The model under review builds one solid part; all positions refer to its coordinate system, in mm. A direction names the side the tool comes from. Coordinates: 2 decimals unless noted, no trailing zeros. Order: outer loops, then holes, each group sorted by start corner. A loop starts at its lowest first (then second) coordinate and runs counter-clockwise, first axis right, second up. Notation, with made-up numbers: (-29, 37) -> (6, 37) arc R19 ccw to (6, 45) -> close; hole circle Ø2 at (1, -25.5). An arc over 180 degrees is marked (long way). Put each result on its own line as item: value.
from build123d import *

# Parameters (mm, degrees)
SKETCH1_R           = 26.5
BOSS_EXTRUDE1_DEPTH = 3
BOSS_EXTRUDE2_START = 3
SKETCH1_3_R         = 26.5
SKETCH1_3_R_2       = 25
BOSS_EXTRUDE2_DEPTH = 10
CUT_EXTRUDE1_DEPTH  = 39.787884706
SKETCH3_R           = 26.5
SKETCH3_R_2         = 25
BOSS_EXTRUDE3_DEPTH = 10
SKETCH5_R           = 0.925
BOSS_EXTRUDE5_DEPTH = 4
FILLET1_R           = 4
CUT_EXTRUDE2_DEPTH  = 44


with BuildPart() as part:
    # Sketch1 → Boss-Extrude1 (new body)
    with BuildSketch(Plane(origin=(0, 0, 0), x_dir=(1, 0, 0), z_dir=(0, 1, 0))):
        with Locations(Location((0, 0, 0), (0, 0, 270))):
            Circle(SKETCH1_R)
    extrude(amount=BOSS_EXTRUDE1_DEPTH)

    # Sketch1<3> → Boss-Extrude2 (add)
    with BuildSketch(Plane(origin=(0, 0, 0), x_dir=(1, 0, 0), z_dir=(0, 1, 0)).offset(BOSS_EXTRUDE2_START)):
        with Locations(Location((0, 0, 0), (0, 0, 270))):
            Circle(SKETCH1_3_R)
        with Locations(Location((0, 0, 0), (0, 0, 270))):
            Circle(SKETCH1_3_R_2, mode=Mode.SUBTRACT)
    extrude(amount=BOSS_EXTRUDE2_DEPTH)

    # Sketch2 → Cut-Extrude1 (cut, through all)
    with BuildSketch(Plane(origin=(0, 3, 0), x_dir=(1, 0, 0), z_dir=(0, 1, 0))):
        with BuildLine():
            ThreePointArc((11.875, 14.831870246), (0, 19), (-11.875, 14.831870246))
            ThreePointArc((-11.875, 14.831870246), (-12.341874249, 10.614995997), (-8.125, 10.148121747))
            ThreePointArc((-8.125, 10.148121747), (0, 13), (8.125, 10.148121747))
            ThreePointArc((8.125, 10.148121747), (12.341874249, 10.614995997), (11.875, 14.831870246))
        make_face()
        with BuildLine():
            ThreePointArc((11.875, -14.831870246), (0, -19), (-11.875, -14.831870246))
            ThreePointArc((-11.875, -14.831870246), (-12.341874249, -10.614995997), (-8.125, -10.148121747))
            ThreePointArc((-8.125, -10.148121747), (0, -13), (8.125, -10.148121747))
            ThreePointArc((8.125, -10.148121747), (12.341874249, -10.614995997), (11.875, -14.831870246))
        make_face()
    extrude(amount=-CUT_EXTRUDE1_DEPTH, mode=Mode.SUBTRACT)

    # Sketch3 → Boss-Extrude3 (add)
    # profile 1 of 5: a face of its own
    with BuildSketch(Plane(origin=(0, 13, 0), x_dir=(1, 0, 0), z_dir=(0, 1, 0))):
        with Locations(Location((0, 0, 0), (0, 0, 270))):
            Circle(SKETCH3_R)
        with Locations(Location((0, 0, 0), (0, 0, 115.041695193))):
            Circle(SKETCH3_R_2, mode=Mode.SUBTRACT)
    # profile 2 of 5: a face of its own
    with BuildSketch(Plane(origin=(0, 13, 0), x_dir=(1, 0, 0), z_dir=(0, 1, 0))):
        with BuildLine():
            ThreePointArc((-10.581942166, 22.65), (-25, 0), (-10.581942166, -22.65))
            Line((-10.581942166, -22.65), (-10.581942166, -20.139140995))
            ThreePointArc((-10.581942166, -20.139140995), (-22.75, 0), (-10.581942166, 20.139140995))
            Line((-10.581942166, 20.139140995), (-10.581942166, 22.65))
        make_face()
    # profile 3 of 5: a face of its own
    with BuildSketch(Plane(origin=(0, 13, 0), x_dir=(1, 0, 0), z_dir=(0, 1, 0))):
        with BuildLine():
            ThreePointArc((10.581942166, 22.65), (0, 25), (-10.581942166, 22.65))
            Line((-10.581942166, 22.65), (-2.130727575, 22.65))
            ThreePointArc((-2.130727575, 22.65), (0, 22.75), (2.130727575, 22.65))
            Line((2.130727575, 22.65), (10.581942166, 22.65))
        make_face()
    # profile 4 of 5: a face of its own
    with BuildSketch(Plane(origin=(0, 13, 0), x_dir=(1, 0, 0), z_dir=(0, 1, 0))):
        with BuildLine():
            Line((10.581942166, -20.139140995), (10.581942166, -22.65))
            ThreePointArc((10.581942166, -22.65), (21.089672285, -13.424817426), (25, 0))
            ThreePointArc((25, 0), (21.089672285, 13.424817426), (10.581942166, 22.65))
            Line((10.581942166, 22.65), (10.581942166, 20.139140995))
            ThreePointArc((10.581942166, 20.139140995), (19.471796069, 11.7648484), (22.75, 0))
            ThreePointArc((22.75, 0), (19.471796069, -11.7648484), (10.581942166, -20.139140995))
        make_face()
    # profile 5 of 5: a face of its own
    with BuildSketch(Plane(origin=(0, 13, 0), x_dir=(1, 0, 0), z_dir=(0, 1, 0))):
        with BuildLine():
            Line((-2.130727575, -22.65), (-10.581942166, -22.65))
            ThreePointArc((-10.581942166, -22.65), (0, -25), (10.581942166, -22.65))
            Line((10.581942166, -22.65), (2.130727575, -22.65))
            ThreePointArc((2.130727575, -22.65), (0, -22.75), (-2.130727575, -22.65))
        make_face()
    extrude(amount=BOSS_EXTRUDE3_DEPTH)

    # Sketch5 → Boss-Extrude5 (add)
    with BuildSketch(Plane(origin=(0, 3, -3), x_dir=(1, 0, 0), z_dir=(0, -1, 0))):
        with Locations(Location((-21.225, 11.76, 0), (0, 0, 90))):
            Circle(SKETCH5_R)
        with Locations(Location((21.225, 11.76, 0), (0, 0, 90))):
            Circle(SKETCH5_R)
        with Locations(Location((-21.225, -5.76, 0), (0, 0, 90))):
            Circle(SKETCH5_R)
        with Locations(Location((21.225, -5.76, 0), (0, 0, 90))):
            Circle(SKETCH5_R)
    extrude(amount=-BOSS_EXTRUDE5_DEPTH)

    # Fillet1
    fillet1_edges = [part.edges().sort_by_distance(p)[0] for p in [
        (0, 0, -26.5),
    ]]
    fillet(fillet1_edges, radius=FILLET1_R)

    # Sketch6 → Cut-Extrude2 (cut)
    with BuildSketch(Plane(origin=(0, 0, 0), x_dir=(0, 0, -1), z_dir=(1, 0, 0))):
        with BuildLine():
            Line((-3, 19), (3, 19))
            ThreePointArc((3, 19), (7, 15), (3, 11))
            Line((3, 11), (-3, 11))
            ThreePointArc((-3, 11), (-7, 15), (-3, 19))
        make_face()
    extrude(amount=-CUT_EXTRUDE2_DEPTH, mode=Mode.SUBTRACT)


solid = part.part
Item 1: Consider section B-B on z = 12. Count the separate pieces of the cut face and the enclosed holes in it, and give its area (3 significant figures).
Answers below:
separate pieces: 3
enclosed holes: 0
area: 206 mm^2
Item 2: For line 1 (X direction, y = 9, z = 0); line 2 (Y direction, x = -3, z = -1); line 3 (X direction, y = 2.75, z = -14), list the stretches that pass through material, from the lowest coordinate up. Write a range as from..to.
Answers below:
line 1: -26.5..-25, 25..26.5
line 2: 0..3
line 3: -22.26..-12.59, 12.59..22.26
Item 3: For pin 1 Ø9.5 at (x, y) = (-5.5, 17.5) entering from -Z; pin 2 Ø1.9 at (x, z) = (1.5, 24) entering from -Y; pin 3 Ø2 at (y, z) = (16, -21) entering from -X, all flat-tipped, find the tip position at first contact; note any pin that passes through.
Answers below:
pin 1: z = -26.49
pin 2: y = 0.04
pin 3: x = -17.39
Item 4: Mouldability with a two-part tool opening along Z and no side actions: class faces 1 (the cylindrical face through (12.3, 1.521, -10.564)), 2 (the flat face through (0, 0, 0)) as +Z half, -Z half, draft (parallel to the pull), parting line (faces both ways), or undercut.
Answers below:
face 1: undercut
face 2: draft
Item 5: For faces 3 (the flat face through (-26, 11, 0)), 4 (the cylindrical face through (0, 2, 19)), 5 (the cylindrical face through (21.08, 7.93, 13.44)), 6 (the flat face through (-10.582, 18, -21)), list the 3-axis set-ups (+Z, -Z, +X, -X, +Y, -Y) from which the entire face can be reached by the end or side of a thin tool; tool diameter is ignored.
Answers below:
face 3: -X
face 4: +Y, -Y
face 5: none
face 6: +Y
Item 6: Consider section A-A on y = 5. Write out the cut boundary in (x, z) (3 decimals).
Answers below:
outline: circle Ø53 at (0, 0); circle Ø1.85 at (-21.225, -8.76); circle Ø1.85 at (-21.225, 8.76); circle Ø1.85 at (21.225, -8.76); circle Ø1.85 at (21.225, 8.76); hole circle Ø50 at (0, 0)
Item 7: Consider section C-C on y = 2.25. Write out the cut boundary in (x, z) (3 decimals).
Answers below:
outline: circle Ø52.194 at (0, 0); hole (-11.875, -14.832) arc R19 ccw to (11.875, -14.832) arc R3 ccw to (8.125, -10.148) arc R13 cw to (-8.125, -10.148) arc R3 ccw to start; hole (-11.875, 14.832) arc R3 ccw to (-8.125, 10.148) arc R13 cw to (8.125, 10.148) arc R3 ccw to (11.875, 14.832) arc R19 ccw to start
